Work out the finished part from the listing and answer in its coordinate system (mm). Face numbers are marked on the shaded views. A direction names the side the tool comes from. Coordinates: 2 decimals unless noted, no trailing zeros. Write each loop counter-clockwise with the first axis right and the second up, starting at its lowest first coordinate (ties: lowest second). Pieces come first, ordered by that corner, then holes. Notation, with made-up numbers: (-7.5, 36.5) - (24.5, 36.5) arc R15 ccw to (24.5, 50.5) - close; hole circle Ø1 at (-31.75, -13.5). An arc over 180 degrees is marked (long way). Use a Markdown table: item, result. Add a question column.
(1) The part is cut by section A-A, the plane z = -20. Give the vertices of the cut face in (x, y), then the cut area to 3 significant figures.
(2) Find the intervals of material crossed by line 1 (Z direction, x = -11.5, y = 1.1); line 2 (Y direction, x = -13, z = -83); line 3 (Z direction, x = -13.25, y = -2.25), in increasing order. Write a range as from..to.
(3) The part is cut by section C-C, the plane x = -2.25. Give the vertices of the cut face in (y, z).
(4) A tool of negligible diameter and unlimited length cuts with its end or side. For the marked faces 1, 2 and 3, from which of +Z, -Z, +X, -X, +Y, -Y can it reach the whole face along a straight path? Write none if from no direction.
(5) The part is cut by section B-B, the plane x = -11.5. Give the vertices of the cut face in (y, z).
(6) Given pin 1 Ø5 at (x, z) = (-11.5, -218.782) entering from -Y; pin 2 Ø3 at (x, z) = (-11.5, -20) entering from -Y, each flat-ended and moving along its own axis, determine where each tip first touches the part or whether it passes through.
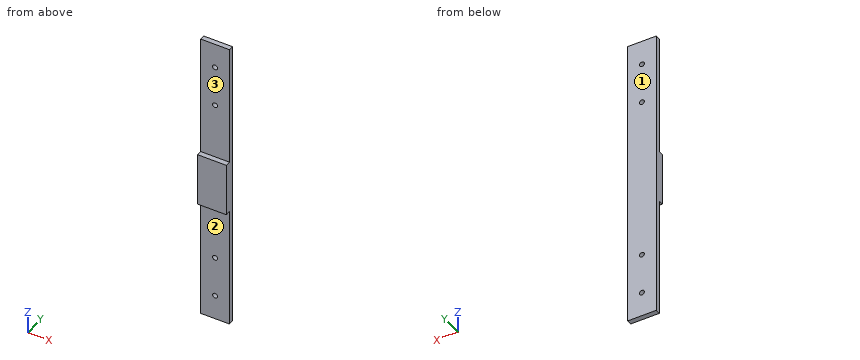
Autodesk Inventor part; units mm, degrees
ref_plane "YZ Plane" through (0, 0, 0) normal (1, 0, 0) x (0, 1, 0)
ref_plane "XZ Plane" through (0, 0, 0) normal (0, 1, 0) x (-1, 0, 0)
ref_plane "XY Plane" through (0, 0, 0) normal (0, 0, 1) x (1, 0, 0)
sketch "Sketch1" plane through (0, 0, 0) normal (0, 1, 0) x (-1, 0, 0)
  line L0 (23, 0) -> (0, 0)
  line L1 (0, 0) -> (0, -238.782)
  line L2 (0, -238.782) -> (23, -238.782)
  line L3 (23, -238.782) -> (23, 0)
  dimension "d2" = 238.782
extrude "Extrusion1" add sketch "Sketch1" along normal blind 4
sketch "Sketch3" plane through (0, 0, 0) normal (0, -1, 0) x (1, 0, 0)
  line L0 (0, 0) -> (0, -238.782)
  line L1 (0, -119.391) -> (0, -136.891)
  line L2 (0, -136.891) -> (0, -101.891)
  line L3 (0, -101.891) -> (-23, -101.891)
  line L4 (-23, -238.782) -> (-23, 0)
  line L5 (-23, -101.891) -> (-23, -136.891)
  line L6 (0, -136.891) -> (-23, -136.891)
  dimension "d5" = 17.5
  dimension "d6" = 35
extrude "Extrusion2" add sketch "Sketch3" along normal blind 4.15
sketch "Sketch4" plane through (0, 0, 0) normal (0, -1, 0) x (1, 0, 0)
  circle A0 centre (-11.5, -185.782) radius 2
  circle A1 centre (-11.5, -218.782) radius 2
  circle A2 centre (-11.5, -20) radius 2
  circle A3 centre (-11.5, -53) radius 2
  point P0 (0, 0)
extrude "Extrusion3" cut sketch "Sketch4" against normal up to surface (4 mm away)
sketch "Sketch5" plane through (-23, 0, -101.891) normal (0, 0, 1) x (1, 0, 0)
  line L0 (0, 0) -> (23, 0)
  line L1 (0, 0) -> (0, -4.15)
  line L2 (23, -4.15) -> (0, -4.15)
  line L3 (23, 0) -> (23, -4.15)
  point P0 (23, 0)
extrude "Extrusion4" add sketch "Sketch5" along normal blind 4
sketch "Sketch6" plane through (0, 0, -136.891) normal (0, 0, -1) x (-1, 0, 0)
  line L0 (0, 0) -> (23, 0)
  line L1 (0, 0) -> (0, -4.15)
  line L2 (23, -4.15) -> (0, -4.15)
  line L3 (23, 0) -> (23, -4.15)
extrude "Extrusion5" add sketch "Sketch6" along normal blind 4
properties part number "battery_support"
Model answer:
| question | item | result |
|---|---|---|
| 1 | outline | (-23, 0) - (-13.5, 0) - (-13.5, 4) - (-23, 4) - close; (-9.5, 0) - (0, 0) - (0, 4) - (-9.5, 4) - close |
| 1 | area | 76.0 mm^2 |
| 2 | line 1 | -238.78..-220.78, -216.78..-187.78, -183.78..-55, -51..-22, -18..0 |
| 2 | line 2 | 0..4 |
| 2 | line 3 | -140.89..-97.89 |
| 3 | outline | (-4.15, -140.89) - (0, -140.89) - (0, -238.78) - (4, -238.78) - (4, 0) - (0, 0) - (0, -97.89) - (-4.15, -97.89) - close |
| 4 | face 1 | +Z, -Z, +X, -X, +Y |
| 4 | face 2 | -Z, +X, -X, -Y |
| 4 | face 3 | +Z, +X, -X, -Y |
| 5 | outline | (-4.15, -140.89) - (0, -140.89) - (0, -183.78) - (4, -183.78) - (4, -55) - (0, -55) - (0, -97.89) - (-4.15, -97.89) - close; (0, -238.78) - (4, -238.78) - (4, -220.78) - (0, -220.78) - close; (0, -216.78) - (4, -216.78) - (4, -187.78) - (0, -187.78) - close; (0, -51) - (4, -51) - (4, -22) - (0, -22) - close; (0, -18) - (4, -18) - (4, 0) - (0, 0) - close |
| 6 | pin 1 | y = 0 |
| 6 | pin 2 | through |
